The listing builds one solid part. Answer for the finished solid, in the listing's coordinates (mm). A direction names the side the tool comes from. Round coordinates to 2 decimals unless told otherwise and drop trailing zeros. Write each loop counter-clockwise with the first axis right and the second up, starting at its lowest first coordinate (ties: lowest second). Pieces come first, ordered by that corner, then holes. Notation, with made-up numbers: (-34, 84.5) - (-22, 84.5) arc R36 ccw to (-22, 122.5) - close; hole circle Ø6 at (-37.5, 30). An arc over 180 degrees is marked (long way). Answer as CSV lines item,"result". Start each with the question number.
Item 1: A cutting plane is placed at D-D on y = 8.75. Determine the outline of the cut face in (x, z).
Item 2: A cutting plane is placed at A-A on x = -6.25. Determine the outline of the cut face in (y, z).
Item 3: For a pull along Z with two mould halves and no side action, classify faces 6 (the flat face through (10.74, 0.46, 16.91)), 7 (the cylindrical face through (0.243, 3.665, 8.106)), 8 (the flat face through (-14, 3, 6)), 9 (the flat face through (2.953, 0.516, 7.193)) as pulls with the +Z half, pulls with the -Z half, needs draft (parallel to the pull), parting line crosses it, or undercut.
Item 4: A cutting plane is placed at C-C on x = 8. Determine the outline of the cut face in (y, z).
Item 5: Straight lines are drawn through the part: line 1 along Z through (x, y) = (10.75, -5.25); line 2 along X through (y, z) = (3.75, 15.75); line 3 along Z through (x, y) = (-5.75, -1). For each, find the intervals that lie inside material, in ascending order. Write a range as [from, to].
Item 6: Flat-ended cylindrical pins translate along their axes: pin 1 (1.5 mm diameter, centred on y = -3.5, z = 16.5, fed in from -X); pin 2 (2 mm diameter, centred on x = 10, y = -6, fed in from -Z); pin 3 (1.2 mm diameter, centred on x = -13.5, z = 10, fed in from -Y); pin 4 (6 mm diameter, centred on x = 0, z = 9.5, fed in from -Y). Find the tip coordinate at first contact, or state that the pin passes through.
Item 7: Which of the six approach directions +Z, -Z, +X, -X, +Y, -Y give full straight-line access (tool end or side, diameter ignored) to faces 1 (the flat face through (-10.74, 0.46, 16.91)), 2 (the flat face through (-7, -1.9, 19.1)), 3 (the flat face through (-13, 2, 7)), 4 (the flat face through (0.196, -4.441, 3.023)), 5 (the flat face through (13, -2, 2))?
Item 8: A cutting plane is placed at B-B on z = 2. Determine the outline of the cut face in (x, y).
```python
from build123d import *

# Parameters (mm, degrees)
F0_W      = 28
F0_H      = 20
F1_DEPTH  = 20
F3_DEPTH  = 20
F6_DEPTH  = 17.5
F7_W      = 1.5
F7_H      = 4
F8_DEPTH  = 40
F12_DEPTH = 15
F15_D     = 14.5
F17_DEPTH = 20
F19_DEPTH = 12.5


with BuildPart() as f1:
    # F0 (on Top) → F1 (new body)
    with BuildSketch(Plane.XY):
        Rectangle(F0_W, F0_H)
    extrude(amount=F1_DEPTH)


with BuildPart() as f3:
    # F2 (on Top) → F3 (new body)
    with BuildSketch(Plane.XY):
        Polygon((-14, 3.5), (-7.5, 10), (-14, 10), align=None)
    extrude(amount=F3_DEPTH)


with BuildPart() as f4_1:
    # F4: instance of F3
    add(f3.part.mirror(Plane.YZ))


with BuildPart() as f6:
    # F5 (on Right) → F6 (new body, symmetric)
    with BuildSketch(Plane.YZ):
        Polygon((-0.083567, 27.704372), (10, 0), (10, 27.704372), align=None)
    extrude(amount=F6_DEPTH, both=True)


with BuildPart() as f8:
    # F7 (on Top) → F8 (new body)
    with BuildSketch(Plane.XY):
        with Locations((-13.25, 0)):
            Rectangle(F7_W, F7_H)
    extrude(amount=F8_DEPTH)


with BuildPart() as f9_1:
    # F9: instance of F8
    add(f8.part.mirror(Plane.YZ))


with BuildPart() as f1_1:
    add(f1.part)

    # F10: cut F3, F4_1, F6, F8, F9_1
    add(f3.part, mode=Mode.SUBTRACT)
    add(f4_1.part, mode=Mode.SUBTRACT)
    add(f6.part, mode=Mode.SUBTRACT)
    add(f8.part, mode=Mode.SUBTRACT)
    add(f9_1.part, mode=Mode.SUBTRACT)


with BuildPart() as f12:
    # F11 (on Right) → F12 (new body, symmetric)
    with BuildSketch(Plane.YZ):
        Polygon((-10, 36.085653), (-10, 1), (1.276311, 5.104242), align=None)
    extrude(amount=F12_DEPTH, both=True)


with BuildPart() as f1_2:
    add(f1_1.part)

    # F13: cut F12
    add(f12.part, mode=Mode.SUBTRACT)

    # F15 (through all)
    with Locations(Plane(origin=(0, 2.767483, 1.007281), x_dir=(1, 0, 0), z_dir=(0, -0.939693, -0.34202))):
        with Locations((0, 13.609894)):
            Hole(F15_D / 2)


with BuildPart() as f17:
    # F16 (on Right) → F17 (new body, symmetric)
    with BuildSketch(Plane.YZ):
        Polygon((-6.932441, 16.194142), (0, 20.196589), (-9.243255, 20.196589), align=None)
    extrude(amount=F17_DEPTH, both=True)


with BuildPart() as f19:
    # F18 (on face) → F19 (new body, symmetric)
    with BuildSketch(Plane(origin=(0, 8.830222, 3.213938), x_dir=(-1, 0, 0), z_dir=(0, 0.939693, 0.34202))):
        Polygon((14, 26.39773), (4, 26.39773), (14, 10.579799), align=None)
    extrude(amount=F19_DEPTH, both=True)


with BuildPart() as f20_1:
    # F20: instance of F19
    add(f19.part.mirror(Plane.YZ))


with BuildPart() as f1_3:
    add(f1_2.part)

    # F21: cut F20_1, F19, F17
    add(f20_1.part, mode=Mode.SUBTRACT)
    add(f19.part, mode=Mode.SUBTRACT)
    add(f17.part, mode=Mode.SUBTRACT)


solid = f1_3.part
```
Geometry says:
1,outline,"(-8.75, 0) - (8.75, 0) - (8.75, 3.43) - (-8.75, 3.43) - close"
2,outline,"(-10, 0) - (10, 0) - (5.43, 12.55) - (-0.63, 10.34) - (1.28, 5.1) - (-10, 1) - close; (-3.48, 18.18) - (-3.14, 17.25) - (2.92, 19.46) - (2.72, 20) - (-0.34, 20) - close"
3,face 6,"pulls with the +Z half"
3,face 7,"undercut"
3,face 8,"needs draft"
3,face 9,"undercut"
4,outline,"(-10, 0) - (9.5, 0) - (9.5, 1.37) - (2.72, 20) - (-0.34, 20) - (-3.48, 18.18) - (1.28, 5.1) - (-10, 1) - close"
5,line 1,"z = [0, 2.73]"
5,line 2,"x = [-12.14, -7.25], [7.25, 12.14]"
5,line 3,"z = [0, 4.28], [18.82, 19.62]"
6,pin 1,"stops at x = -10.42"
6,pin 2,"stops at z = 0"
6,pin 3,"stops at y = 2"
6,pin 4,"stops at y = 0.5"
7,face 1,"+Z, -X, -Y"
7,face 2,"+Z, +X, -X, -Y"
7,face 3,"+Z, -Z, -X"
7,face 4,"+X, -X, -Y"
7,face 5,"+Z, -Z, +X"
8,outline,"(-14, -7.25) - (14, -7.25) - (14, -2) - (12.5, -2) - (12.5, 2) - (14, 2) - (14, 3.5) - (8.23, 9.27) - (-8.23, 9.27) - (-14, 3.5) - (-14, 2) - (-12.5, 2) - (-12.5, -2) - (-14, -2) - close"
